Geometry: final body of the model. Coordinates: model frame, mm. A direction names the side the tool comes from. Give positions to 0.01 mm unless a question says otherwise; leave off trailing zeros. Loops run counter-clockwise (first coordinate to the right, second up) from the corner with the lowest first, then second, coordinate; pieces in that order, holes last. Notation, with made-up numbers: (2.25, 13) -> (8.25, 13) arc R33 cw to (8.25, 52) -> close; hole circle Ø9 at (40, 12). An arc over 180 degrees is marked (long way). One line per question, with ' | ' between items. Start each with the question number.
Item 1: Mould query, pull axis X, two halves, no side actions, for faces 5 (the flat face through (-37, 7, -5)), 6 (the flat face through (-2.529, 34, 3)), 7 (the cylindrical face through (2.15, 37.12, -4.02)), 8 (the cylindrical face through (3.58, 37.93, -4.86)). Classes: released by +X, released by -X, zero draft, split by the parting line, or undercut.
Item 2: Set-up query: faces 1 (the flat face through (4.991, 23, 19)), 2 (the cylindrical face through (-5.44, 7.46, -2.48)), 3 (the flat face through (-1, 39, 6.448)), 4 (the flat face through (1, 22, 18.448)). Return all of +Z, -Z, +X, -X, +Y, -Y with unobstructed straight access to the full face (end or side cutting, diameter ignored); none if empty.
Item 3: Section C-C on y = 3.5. Return loops of the section in (x, z).
Item 4: Pin query (flat end, axial travel): P1, Ø1.5, axis at x = -13.5, z = -3.5, coming from the -Y side; P2, Ø1.5, axis at x = -34, y = 7.5, coming from the -Z side; P3, Ø1.7, axis at y = 37.5, z = 2.5, coming from the +X side; P4, Ø7.5, axis at y = 7, z = -1, coming from the +X side. Return the tip coordinate at first contact, or that it passes through.
Item 5: Section A-A on y = 30. Return loops of the section in (x, z).
Item 6: Section B-B on x = -4.5. Return loops of the section in (y, z).
Item 7: Material intervals for line 1 along Z through (x, y) = (-21, 5.5); line 2 along X through (y, z) = (33.5, 6); line 3 along Y through (x, z) = (-12.5, -3.5), sorted ascending. Write a range as [from, to].
Item 8: Section D-D on x = -50. Return loops of the section in (y, z).
Autodesk Inventor part; units mm, degrees
ref_plane "YZ Plane" through (0, 0, 0) normal (1, 0, 0) x (0, 1, 0)
ref_plane "XZ Plane" through (0, 0, 0) normal (0, 1, 0) x (-1, 0, 0)
ref_plane "XY Plane" through (0, 0, 0) normal (0, 0, 1) x (1, 0, 0)
sketch "Sketch1" plane through (0, 0, 0) normal (0, 1, 0) x (-1, 0, 0)
  circle A0 centre (0, 0) radius 12.5
  line L0 (0, 0) -> (7.75, 0) construction
  circle A1 centre (5.4801, -5.4801) radius 2
  circle A2 centre (-5.4801, -5.4801) radius 2
  circle A3 centre (-5.4801, 5.4801) radius 2
  circle A4 centre (5.4801, 5.4801) radius 2
  circle A5 centre (0, -7.75) radius 2
  circle A6 centre (0, 7.75) radius 2
  dimension "d0" = 25
  dimension "d3" = 4
  dimension "d6" = 360
  dimension "d8" = 4
  dimension "d11" = 360
extrude "Extrusion1" add sketch "Sketch1" along normal blind 5
sketch "Sketch2" plane through (0, 5, 0) normal (0, 1, 0) x (1, 0, 0)
  line L0 (4.991, -3.5408) -> (4.991, 3.5408)
  line L1 (-66.4503, 5) -> (-66.4503, -5)
  line L2 (4.991, -4.9385) -> (14.991, -4.9385) construction
  line L3 (-82.7386, 0) -> (31.2793, 0)
  arc A0 (-3.5548, -4.9385) -> (-7.4216, -5) centre (-5.4801, -5.4801) ccw
  line L4 (-66.4503, -5) -> (-7.4216, -5)
  line L5 (-3.5548, -4.9385) -> (3.5548, -4.9385)
  circle A1 centre (-5.4801, 5.4801) radius 2
  arc A2 (-7.4216, 5) -> (-3.5497, 4.9571) centre (-5.4801, 5.4801) ccw
  line L6 (3.5497, 4.9571) -> (-3.5497, 4.9571)
  line L7 (-7.4216, 5) -> (-66.4503, 5)
  arc A3 (4.991, -3.5408) -> (3.5548, -4.9385) centre (5.4801, -5.4801) ccw
  circle A4 centre (5.4801, 5.4801) radius 2
  arc A5 (3.5497, 4.9571) -> (4.991, 3.5408) centre (5.4801, 5.4801) ccw
  dimension "d24" = 10
  dimension "d25" = 90
  dimension "d26" = 70
  dimension "d27" = 4
  dimension "d28" = 4
  dimension "d29" = 4
  dimension "d30" = 4
extrude "Extrusion2" add sketch "Sketch2" along normal blind 5 contours A3 L5 A0 L4 L1 L3 L0 | L3 L1 L7 A1 L6 A4 L0
sketch "Sketch4" plane through (0, 10, 0) normal (0, 1, 0) x (1, 0, 0)
  line L0 (-3.5548, -4.9385) -> (3.5548, -4.9385)
  line L1 (-3.5548, -4.9385) -> (3.5548, -4.9385)
  line L2 (3.5497, 4.9571) -> (-3.5497, 4.9571)
  line L3 (-3.5497, 4.9571) -> (3.5497, 4.9571)
  line L4 (-4.4956, -10.2074) -> (2.6201, -10.2074)
  point P0 (0, 0)
sketch "Sketch8" plane through (0, 5, 0) normal (0, 1, 0) x (1, 0, 0)
  circle A0 centre (-5.4801, 5.4801) radius 2
  circle A1 centre (-5.4801, 5.4801) radius 3
  circle A2 centre (-5.4801, -5.4801) radius 2
  circle A3 centre (-5.4801, -5.4801) radius 3
  circle A4 centre (5.4801, 5.4801) radius 2
  circle A5 centre (5.4801, 5.4801) radius 3
  arc A6 (3.5548, -4.9385) -> (4.991, -3.5408) centre (5.4801, -5.4801) ccw
  circle A7 centre (5.4801, -5.4801) radius 3
  point P0 (0, 0)
  dimension "d50" = 6
  dimension "d51" = 6
  dimension "d52" = 6
  dimension "d53" = 6
extrude "Extrusion6" cut sketch "Sketch8" along normal blind 39.25 contours A0 | A1 | A2 | A3 | A4 | A5 | A7
sketch "Sketch30" plane through (0, 10, 0) normal (0, 1, 0) x (1, 0, 0)
  line L0 (-2.5294, -4.9385) -> (2.5294, -4.9385)
  arc A0 (-8.4414, 5) -> (-2.526, 4.9571) centre (-5.4801, 5.4801) ccw
  line L1 (-2.5294, -18.4485) -> (-2.5294, 18.5515)
  arc A1 (4.991, -2.5202) -> (2.5294, -4.9385) centre (5.4801, -5.4801) ccw
  arc A2 (2.526, 4.9571) -> (4.991, 2.5202) centre (5.4801, 5.4801) ccw
  point P0 (0, 0)
  dimension "d90" = 13.51
  dimension "d91" = 37
sketch "Sketch31" plane through (4.991, 5, 2.5202) normal (1, 0, 0) x (0, 0, -1)
  point P0 (2.5202, -5)
ref_plane "Work Plane4" through (-2.5294, 10, 18.4485) normal (1, 0, 0) x (0, 0, -1)
sketch "Sketch41" plane through (-2.5294, 10, 18.4485) normal (1, 0, 0) x (0, 0, -1)
  line L0 (0, 0) -> (-2, 0)
  line L1 (-2, 0) -> (39, 0)
  line L2 (15.9283, 0) -> (20.9687, 0)
  line L3 (39, 0) -> (39, 25)
  line L4 (-2, 25) -> (-2, 0)
  line L5 (18.5, 1.9993) -> (0, 1.9993)
  line L6 (18.5, 1.9993) -> (37, 1.9993)
  line L7 (0, 1.9993) -> (37, 1.9993)
  line L8 (37, 23) -> (37, 1.9993)
  line L9 (0, 12.5) -> (0, 23)
  line L10 (0, 23) -> (0, 1.9993)
  line L11 (17, 23) -> (17, 33)
  line L12 (17, 33) -> (12, 33)
  line L13 (12, 33) -> (12, 25)
  line L14 (20, 23) -> (20, 33)
  line L15 (20, 33) -> (25, 33)
  line L16 (25, 33) -> (25, 25)
  line L17 (25, 25) -> (39, 25)
  line L18 (39, 25) -> (39, 0)
  line L19 (39, 0) -> (-2, 0)
  line L20 (30.9485, -10) -> (5.9485, -10)
  line L21 (-2, 0) -> (-2, 25)
  line L22 (-2, 25) -> (12, 25)
  line L23 (12, 33) -> (17, 33)
  line L24 (17, 33) -> (17, 23)
  line L25 (17, 23) -> (0, 23)
  line L26 (0, 23) -> (0, 1.9993)
  line L27 (37, 1.9993) -> (0, 1.9993)
  line L28 (30.9485, -5) -> (5.9485, -5)
  line L29 (37, 1.9993) -> (37, 23)
  line L30 (37, 23) -> (20, 23)
  line L31 (20, 23) -> (20, 33)
  line L32 (25, 33) -> (25, 25)
  point P0 (18.4485, -10)
  point P1 (13.4485, -5)
  point P2 (23.4485, -5)
  point P3 (0, 12.5)
  dimension "d129" = 2
  dimension "d130" = 41
  dimension "d131" = 25
  dimension "d132" = 41
  dimension "d138" = 3
  dimension "d139" = 10
  dimension "d140" = 5
  dimension "d141" = 5
extrude "Extrusion14" add sketch "Sketch41" along normal up to surface (7.5204 mm away)
sketch "Sketch42" plane through (-2.5294, 35, 6.4485) normal (0, 0, 1) x (1, 0, 0)
  line L0 (0, 0) -> (0, 8)
  line L1 (7.5204, -2) -> (7.5204, 8)
  line L2 (0, 8) -> (7.5204, 8)
  circle A0 centre (3.7602, 3.8975) radius 2
  point P0 (2.5294, -35)
  dimension "d144" = 4
extrude "Extrusion15" cut sketch "Sketch42" against normal through all
fillet "Fillet3" radius 2 8 edges at (1.2308, 11.9993, 18.4485) (1.2308, 10, 20.4485) (1.2308, 10, -20.5515) (1.2308, 35, -20.5515) (1.2308, 33, -18.5515) (1.2308, 11.9993, -18.5515) (1.2308, 33, 18.4485) (1.2308, 35, 20.4485)
extrude "Extrusion17" cut sketch "Sketch1" along normal through all contours A2 | A3
properties part number "Marker holder"
Result sheet:
1) face 5: zero draft | face 6: released by -X | face 7: undercut | face 8: released by +X
2) face 1: +Z, -Z, +X, +Y | face 2: -Z, +Y | face 3: +Z, +X, -X, +Y | face 4: +X, -X
3) outline: circle Ø25 at (0, 0); hole circle Ø4 at (-5.48, -5.48); hole circle Ø4 at (-5.48, 5.48); hole circle Ø4 at (0, -7.75); hole circle Ø4 at (0, 7.75); hole circle Ø4 at (5.48, -5.48); hole circle Ø4 at (5.48, 5.48)
4) P1: stops at y = 5 | P2: stops at z = -5 | P3: stops at x = 4.99 | P4: stops at x = 12.5
5) outline: (-2.53, -20.55) -> (4.99, -20.55) -> (4.99, -18.55) -> (-2.53, -18.55) -> close; (-2.53, 18.45) -> (4.99, 18.45) -> (4.99, 20.45) -> (-2.53, 20.45) -> close
6) outline: (0, -11.66) -> (5, -11.66) -> (5, -7.22) -> (0, -7.22) -> close; (0, -3.74) -> (5, -3.74) -> (5, -2.64) -> (10, -2.64) -> (10, 2.64) -> (5, 2.64) -> (5, 3.74) -> (0, 3.74) -> close; (0, 7.22) -> (5, 7.22) -> (5, 11.66) -> (0, 11.66) -> close
7) line 1: z = [-5, 5] | line 2: x = [-2.53, 3.55] | line 3: y = [5, 10]
8) outline: (5, -5) -> (10, -5) -> (10, 5) -> (5, 5) -> close
